Read the model definition and answer for the solid it produces. Units are mm, in the model's axes. Face numbers are marked on the shaded views. A direction names the side the tool comes from. Give positions to 0.01 mm unless a question says otherwise; leave off trailing zeros. Order: outer loops, then holes, each group sorted by start corner. A loop starts at its lowest first (then second) coordinate and runs counter-clockwise, first axis right, second up. Notation, with made-up numbers: (-37.5, 25) - (17.5, 25) arc R29 cw to (17.5, 49) - close; hole circle Ø10 at (79.25, 34.25). An arc over 180 degrees is marked (long way). Write item = value, one per line.
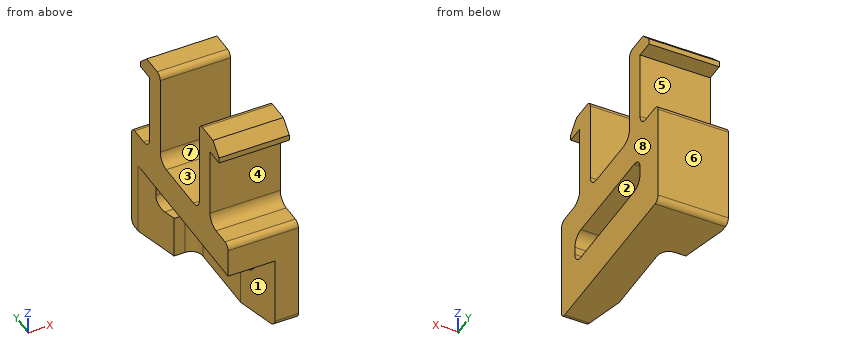
```python
from build123d import *

# Parameters (mm, degrees)
ESQUISSE1_W             = 6
ESQUISSE1_H             = 16
EXTRUSION1_DEPTH        = 3.7
ESQUISSE2_W             = 6
ESQUISSE2_H             = 3
ESQUISSE2_W_2           = 3
ESQUISSE2_H_2           = 2.2
EXTRUSION2_DEPTH        = 2.7
ESQUISSE3_W             = 3
ESQUISSE3_H             = 11
ENL_V_MAT_EXTRU_1_DEPTH = 5
ESQUISSE4_W             = 6
ESQUISSE4_H             = 16
EXTRUSION3_DEPTH        = 3
EXTRUSION4_DEPTH        = 6
CHANFREIN1_SIZE         = 1
CONG_1_R                = 1
CONG_2_R                = 0.5
ENL_V_MAT_EXTRU_2_REACH = 78.526


with BuildPart() as part:
    # Esquisse1 → Extrusion1 (new body)
    with BuildSketch(Plane.XY):
        with Locations((55.8, 37.58978076)):
            Rectangle(ESQUISSE1_W, ESQUISSE1_H)
    extrude(amount=EXTRUSION1_DEPTH)

    # Esquisse2 → Extrusion2 (add)
    with BuildSketch(Plane.XY.offset(3.7)):
        with Locations((55.8, 44.08978076)):
            Rectangle(ESQUISSE2_W, ESQUISSE2_H)
        with Locations((57.3, 30.68978076)):
            Rectangle(ESQUISSE2_W_2, ESQUISSE2_H_2)
    extrude(amount=EXTRUSION2_DEPTH)

    # Esquisse3 → Enlèv. mat.-Extru.1 (cut)
    with BuildSketch(Plane.XY.offset(3.7)):
        with Locations((54.3, 35.08978076)):
            Rectangle(ESQUISSE3_W, ESQUISSE3_H)
    extrude(amount=-ENL_V_MAT_EXTRU_1_DEPTH, mode=Mode.SUBTRACT)

    # Esquisse4 → Extrusion3 (add)
    with BuildSketch(Plane.XY.offset(6.4)):
        with Locations((55.8, 37.58978076)):
            Rectangle(ESQUISSE4_W, ESQUISSE4_H)
    extrude(amount=EXTRUSION3_DEPTH)

    # Esquisse5 → Extrusion4 (add)
    with BuildSketch(Plane.ZY.offset(-52.8)):
        Polygon((8.183216319, 42.58978076), (16.4, 42.58978076), (16.4, 44.08978076), (17.9, 44.08978076), (17.9, 40.83978076), (9.2, 40.83978076), (9.2, 34.33978076), (17.9, 34.33978076), (17.9, 31.08978076), (16.4, 31.08978076), (16.4, 32.58978076), (8.183216319, 32.58978076), align=None)
    extrude(amount=-EXTRUSION4_DEPTH)

    # Chanfrein1
    chanfrein1_edges = [part.edges().sort_by_distance(p)[0] for p in [
        (55.8, 44.08978076, 17.9),
        (55.8, 31.08978076, 17.9),
    ]]
    chamfer(chanfrein1_edges, length=CHANFREIN1_SIZE)

    # Congé1
    cong_1_edges = [part.edges().sort_by_distance(p)[0] for p in [
        (55.8, 40.58978076, 1.85),
        (55.8, 42.58978076, 6.4),
        (55.8, 42.58978076, 3.7),
        (57.3, 31.78978076, 3.7),
        (57.3, 31.78978076, 6.4),
        (55.8, 34.33978076, 9.4),
        (55.8, 42.58978076, 9.4),
        (55.8, 32.58978076, 9.4),
        (55.8, 40.83978076, 9.4),
    ]]
    fillet(cong_1_edges, radius=CONG_1_R)

    # Congé2
    cong_2_edges = [part.edges().sort_by_distance(p)[0] for p in [
        (57.3, 29.58978076, 0),
        (55.8, 45.58978076, 0),
        (55.8, 29.58978076, 9.4),
        (55.8, 45.58978076, 9.4),
        (55.8, 40.83978076, 17.9),
        (55.8, 34.33978076, 17.9),
    ]]
    fillet(cong_2_edges, radius=CONG_2_R)

    # Enlèv. mat.-Extru.2: up to this face of the body (flat: up to its plane)
    enl_v_mat_extru_2_end = Plane(part.part.faces().sort_by_distance((55.569230769, 36.266703837, 6.4))[0])
    # Esquisse6 → Enlèv. mat.-Extru.2 (cut, up to the picked face)
    with BuildSketch(Plane(origin=(0, 0, 0), x_dir=(-1, 0, 0), z_dir=(0, 0, -1)), mode=Mode.PRIVATE) as enl_v_mat_extru_2_sk1:
        Polygon((-56.8, 29.58978076), (-52.381825652, 46.078631902), (-52.381825652, 29.58978076), align=None)
    enl_v_mat_extru_2_tool1 = split(extrude(enl_v_mat_extru_2_sk1.sketch, amount=-ENL_V_MAT_EXTRU_2_REACH, mode=Mode.PRIVATE), bisect_by=enl_v_mat_extru_2_end, keep=Keep.BOTH, mode=Mode.PRIVATE)
    add(enl_v_mat_extru_2_tool1.solids().sort_by(Axis((53.85455, 35.086064, 0), (0, 0, 1)))[0], mode=Mode.SUBTRACT)


solid = part.part
```
1. Section B-B (y = 37.5) is taken. Determine the outline of the cut face in (x, z).
Recorded:
outline = (52.8, 6.4) - (58.8, 6.4) - (58.8, 9.4) - (52.8, 9.4) - close; (55.8, 0) - (58.8, 0) - (58.8, 3.7) - (55.8, 3.7) - close
2. Flat-ended cylindrical pins translate along their axes: pin 1 (1.2 mm diameter, centred on x = 55, y = 44.5, fed in from +Z); pin 2 (1.8 mm diameter, centred on x = 56.5, z = 14, fed in from -Y); pin 3 (1.6 mm diameter, centred on x = 56.5, y = 37, fed in from +Z); pin 4 (5 mm diameter, centred on y = 35, z = 11, fed in from -X). Find the tip coordinate at first contact, or state that the pin passes through.
Recorded:
pin_1 = 17.09
pin_2 = 32.59
pin_3 = 9.4
pin_4 = 52.8
3. Determine the mould class of the marked faces 6, 7 and 8 for opening direction Y: +Y half, -Y half, draft (parallel to the pull), parting line (faces both ways), or undercut.
Recorded:
face_6 = +Y half
face_7 = undercut
face_8 = draft
4. Section C-C (z = 2.25) is taken. Determine the outline of the cut face in (x, y), and give its area (3 significant figures).
Recorded:
outline = (52.8, 44.52) - (53.85, 40.59) - (54.8, 40.59) arc R1 cw to (55.8, 39.59) - (55.8, 33.32) - (56.8, 29.59) - (58.8, 29.59) - (58.8, 45.59) - (52.8, 45.59) - close
area = 59.3 mm^2
5. For the marked faces 1, 2, 3, 4 and 5, determine the directions among +Z, -Z, +X, -X, +Y, -Y from which every point of the face is accessible in a straight line to the end or side of a thin tool.
Recorded:
face_1 = -Z, -X, -Y
face_2 = -X
face_3 = +Z, +X, -X
face_4 = +X, -X, -Y
face_5 = +X, -X, +Y
6. Straight lines are drawn through the part: L1, parallel to Y at x = 55.25, z = 14.25; L2, parallel to Z at x = 55.9, y = 39.75; L3, parallel to Z at x = 54.5, y = 43.75. For each, find the intervals that lie inside material, in ascending order. Write a range as [from, to].
Recorded:
L1 = [32.59, 34.34], [40.84, 42.59]
L2 = [0, 3.7], [6.4, 9.4]
L3 = [0, 9.4], [16.4, 17.24]
7. Section A-A (z = 5) is taken. Determine the outline of the cut face in (x, y), and give its area (3 significant figures).
Recorded:
outline = (52.8, 44.52) - (53.32, 42.59) - (58.8, 42.59) - (58.8, 45.59) - (52.8, 45.59) - close; (56.21, 31.79) - (56.8, 29.59) - (58.8, 29.59) - (58.8, 31.79) - close
area = 22.6 mm^2
